Verification items for the finished model (mm, model axes). A direction names the side the tool comes from. Give positions to 0.01 mm unless a question says otherwise; leave off trailing zeros. Write each loop counter-clockwise with the first axis right and the second up, starting at its lowest first coordinate (ties: lowest second). Pieces come first, ordered by that corner, then holes.
from build123d import *

# Parameters (mm, degrees)
BASISTEIL_MOLDINGFORMUMRELLAV1_0_0_SAK_1_START = 19
BASISTEIL_MOLDINGFORMUMRELLAV1_0_0_S_2_R       = 1.49
BASISTEIL_MOLDINGFORMUMRELLAV1_0_0_S_2_R_2     = 9.27775
BASISTEIL_MOLDINGFORMUMRELLAV1_0_0_SAK_1_DEPTH = 1
AUFSATZ_LINEAR_AUSTRAGEN1_DEPTH                = 1.85
VERRUNDUNG1_R                                  = 0.5


# Read off the part's stored shape, not the designer's step: Basisteil-MoldingFormUmrellaV1_0_0_SAK-1
with BuildPart() as part:
    # Basisteil-MoldingFormUmrellaV1_0_0_S 2 → Basisteil-MoldingFormUmrellaV1_0_0_SAK-1 (new body)
    with BuildSketch(Plane(origin=(0, 0, 0), x_dir=(1, 0, 0), z_dir=(0, 1, 0)).offset(BASISTEIL_MOLDINGFORMUMRELLAV1_0_0_SAK_1_START)):
        with BuildLine():
            Line((5, 15), (-5, 15))
            ThreePointArc((-5, 15), (-12.071067812, 12.071067812), (-15, 5))
            Line((-15, 5), (-15, -5))
            ThreePointArc((-15, -5), (-12.071067812, -12.071067812), (-5, -15))
            Line((-5, -15), (5, -15))
            ThreePointArc((5, -15), (12.071067812, -12.071067812), (15, -5))
            Line((15, -5), (15, 5))
            ThreePointArc((15, 5), (12.071067812, 12.071067812), (5, 15))
        make_face()
        with Locations((9.718159066, -9.341055177)):
            Circle(BASISTEIL_MOLDINGFORMUMRELLAV1_0_0_S_2_R, mode=Mode.SUBTRACT)
        with Locations((-9.718159066, 9.341055177)):
            Circle(BASISTEIL_MOLDINGFORMUMRELLAV1_0_0_S_2_R, mode=Mode.SUBTRACT)
        Circle(BASISTEIL_MOLDINGFORMUMRELLAV1_0_0_S_2_R_2, mode=Mode.SUBTRACT)
    extrude(amount=BASISTEIL_MOLDINGFORMUMRELLAV1_0_0_SAK_1_DEPTH)

    # Skizze1 → Aufsatz-Linear austragen1 (add)
    with BuildSketch(Plane(origin=(0, 0, -15), x_dir=(-1, 0, 0), z_dir=(0, 0, -1))):
        Polygon((0, 16.15), (1.861417329, 19.374069389), (-1.861417329, 19.374069389), align=None)
    aufsatz_linear_austragen1 = extrude(amount=-AUFSATZ_LINEAR_AUSTRAGEN1_DEPTH)

    # Spiegeln1: Aufsatz-Linear austragen1 across plane
    add(aufsatz_linear_austragen1.mirror(Plane(origin=(0, 0, 0), x_dir=(1, 0, 0), z_dir=(0, 0, -1))))

    # Verrundung1
    verrundung1_edges = [part.edges().sort_by_distance(p)[0] for p in [
        (0, 16.15, -14.075),
        (0, 16.15, 14.075),
    ]]
    fillet(verrundung1_edges, radius=VERRUNDUNG1_R)


solid = part.part
Item 1: Sectioned sample at B-B on x = 0. Record the cut outline in (y, z).
Answer key:
outline: (16.65, -15) - (20, -15) - (20, -9.28) - (19, -9.28) - (19, -13.15) - (16.65, -13.15) - close; (16.65, 13.15) - (19, 13.15) - (19, 9.28) - (20, 9.28) - (20, 15) - (16.65, 15) - close
Item 2: Sectioned sample at C-C on y = 18.2. Record the cut outline in (x, z).
Answer key:
outline: (-1.18, -15) - (1.18, -15) - (1.18, -13.15) - (-1.18, -13.15) - close; (-1.18, 13.15) - (1.18, 13.15) - (1.18, 15) - (-1.18, 15) - close
Item 3: Scan lines: line 1 along Z through (x, y) = (0, 19.6); line 2 along Y through (x, z) = (8, -8.5). Record each from-to range of solid material in increasing order.
Answer key:
line 1: z = -15 to -9.28, 9.28 to 15
line 2: y = 19 to 20
Item 4: Sectioned sample at A-A on z = 0. Record the cut outline in (x, y).
Answer key:
outline: (-15, 19) - (-9.28, 19) - (-9.28, 20) - (-15, 20) - close; (9.28, 19) - (15, 19) - (15, 20) - (9.28, 20) - close
Item 5: Release check for a two-part mould opening along Z. For faces 1 (the face through (-11.99, 19.49, -12.15)), 2 (the face through (-10.041, 19.493, -7.886)), 3 (the face through (0, 19, 15)) record: released by +Z, released by -Z, zero draft, split by the parting line, or undercut.
Answer key:
face 1: released by -Z
face 2: undercut
face 3: released by +Z
Item 6: Sectioned sample at D-D on x = -13. Record the cut outline in (y, z).
Answer key:
outline: (19, -11) - (20, -11) - (20, 11) - (19, 11) - close
Item 7: Depth check by flat-ended pin: pin 1 (2 mm diameter, centred on x = 4.5, z = -5.5, fed in from +Y); pin 2 (2 mm diameter, centred on y = 19.5, z = 10, fed in from -X); pin 3 (8 mm diameter, centred on x = -6, z = -0.5, fed in from -Y). Enter the tip coordinate at first touch or a pass-through.
Answer key:
pin 1: passes through
pin 2: stops at x = -14.17
pin 3: stops at y = 19
Item 8: Set-up check for faces 4 (the face through (0, 18, -13.15)), 5 (the face through (-12.15, 19.49, 11.99)): record each of +Z, -Z, +X, -X, +Y, -Y from which the full face is reachable in a straight line by a thin tool's end or side.
Answer key:
face 4: +X, -X, -Y
face 5: +Z, -X, +Y, -Y
